```python
from build123d import *

# Parameters (mm, degrees)
SKETCH1_W           = 500
SKETCH1_H           = 200
BOSS_EXTRUDE1_DEPTH = 500
SKETCH2_W           = 500
SKETCH2_H           = 453.889764575
CUT_EXTRUDE1_DEPTH  = 180


with BuildPart() as part:
    # Sketch1 → Boss-Extrude1 (new body)
    with BuildSketch(Plane(origin=(0, 0, 0), x_dir=(1, 0, 0), z_dir=(0, 1, 0))):
        Rectangle(SKETCH1_W, SKETCH1_H)
    extrude(amount=-BOSS_EXTRUDE1_DEPTH)

    # Sketch2 → Cut-Extrude1 (cut)
    with BuildSketch(Plane.XY.offset(100)):
        with Locations((0, -273.055117713)):
            Rectangle(SKETCH2_W, SKETCH2_H)
    extrude(amount=-CUT_EXTRUDE1_DEPTH, mode=Mode.SUBTRACT)


solid = part.part
```
Part model, mm, in its own coordinate system. A direction names the side the tool comes from. Give positions to 0.01 mm unless a question says otherwise; leave off trailing zeros. Write each loop counter-clockwise with the first axis right and the second up, starting at its lowest first coordinate (ties: lowest second). Pieces come first, ordered by that corner, then holes. Notation, with made-up numbers: (61, 70.25) -> (117, 70.25) arc R7 ccw to (117, 75.25) -> close; hole circle Ø1 at (-17.75, 30.25). An arc over 180 degrees is marked (long way). Put each result on its own line as item: value. Start each with the question number.
Item 1: Which spindle directions (+Z, -Z, +X, -X, +Y, -Y) get a long thin tool onto all of the face, cutting with end or side? Do faces 1 (the face through (-3, -270, -80)), 2 (the face through (250, -156, -81)). Say none if no direction does.
Item 2: Cut at B-B (z = 19.5). List the corners of the cut face in (x, y).
Item 3: Pin check, flat tip, straight feed: pin 1 Ø8 at (x, z) = (0.5, -14) entering from -Y. Stop position of the tip, or through.
Item 4: Cut at A-A (x = -61). List the corners of the cut face in (y, z).
Item 5: Wall check: L1, parallel to Y at x = -143.5, z = -60; L2, parallel to Z at x = 147.5, y = -288. Give the ranges that are in metal, low to high. Write a range as [from, to].
Item 6: Cut at C-C (y = -370). List the corners of the cut face in (x, z).
Answer list:
1. face 1: +Z, +X, -X, -Y
1. face 2: +Z, -Z, +X, +Y, -Y
2. outline: (-250, -46.11) -> (250, -46.11) -> (250, 0) -> (-250, 0) -> close
3. pin 1: stops at y = -46.11
4. outline: (-500, -100) -> (0, -100) -> (0, 100) -> (-46.11, 100) -> (-46.11, -80) -> (-500, -80) -> close
5. L1: y = [-46.11, 0]
5. L2: z = [-100, -80]
6. outline: (-250, -100) -> (250, -100) -> (250, -80) -> (-250, -80) -> close
